```python
from build123d import *

# Parameters (mm, degrees)
BOSS_EXTRUDE1_DEPTH = 10
BOSS_EXTRUDE2_START = 36
BOSS_EXTRUDE2_DEPTH = 36
BOSS_EXTRUDE3_START = 10
BOSS_EXTRUDE3_DEPTH = 10
SKETCH4_R           = 2.5
BOSS_EXTRUDE4_DEPTH = 25
SKETCH4_3_R         = 12.7
BOSS_EXTRUDE5_DEPTH = 2
CUT_EXTRUDE1_START  = -15
CUT_EXTRUDE1_DEPTH  = 15


with BuildPart() as part:
    # Sketch1 → Boss-Extrude1 (new body)
    with BuildSketch(Plane(origin=(0, 0, 0), x_dir=(0, 0, -1), z_dir=(1, 0, 0))):
        with BuildLine():
            Line((-20, 26), (-20, 25))
            ThreePointArc((-20, 25), (-21.464466094, 21.464466094), (-25, 20))
            Line((-25, 20), (-26, 20))
            ThreePointArc((-26, 20), (-27.414213562, 19.414213562), (-28, 18))
            Line((-28, 18), (-28, -18))
            ThreePointArc((-28, -18), (-27.414213562, -19.414213562), (-26, -20))
            Line((-26, -20), (-25, -20))
            ThreePointArc((-25, -20), (-21.464466094, -21.464466094), (-20, -25))
            Line((-20, -25), (-20, -26))
            ThreePointArc((-20, -26), (-19.414213562, -27.414213562), (-18, -28))
            Line((-18, -28), (18, -28))
            ThreePointArc((18, -28), (19.414213562, -27.414213562), (20, -26))
            Line((20, -26), (20, -25))
            ThreePointArc((20, -25), (21.464466094, -21.464466094), (25, -20))
            Line((25, -20), (26, -20))
            ThreePointArc((26, -20), (27.414213562, -19.414213562), (28, -18))
            Line((28, -18), (28, 18))
            ThreePointArc((28, 18), (27.414213562, 19.414213562), (26, 20))
            Line((26, 20), (25, 20))
            ThreePointArc((25, 20), (21.464466094, 21.464466094), (20, 25))
            Line((20, 25), (20, 26))
            ThreePointArc((20, 26), (19.414213562, 27.414213562), (18, 28))
            Line((18, 28), (-18, 28))
            ThreePointArc((-18, 28), (-19.414213562, 27.414213562), (-20, 26))
        make_face()
    extrude(amount=-BOSS_EXTRUDE1_DEPTH)

    # Sketch2 → Boss-Extrude2 (add)
    with BuildSketch(Plane(origin=(0, 0, 0), x_dir=(0, 0, -1), z_dir=(1, 0, 0)).offset(BOSS_EXTRUDE2_START)):
        with BuildLine():
            Line((20, -26), (20, -25))
            ThreePointArc((20, -25), (21.464466094, -21.464466094), (25, -20))
            Line((25, -20), (26, -20))
            ThreePointArc((26, -20), (27.414213562, -19.414213562), (28, -18))
            Line((28, -18), (28, 18))
            ThreePointArc((28, 18), (27.414213562, 19.414213562), (26, 20))
            Line((26, 20), (25, 20))
            ThreePointArc((25, 20), (21.464466094, 21.464466094), (20, 25))
            Line((20, 25), (20, 26))
            ThreePointArc((20, 26), (19.414213562, 27.414213562), (18, 28))
            Line((18, 28), (-18, 28))
            ThreePointArc((-18, 28), (-19.414213562, 27.414213562), (-20, 26))
            Line((-20, 26), (-20, 25))
            ThreePointArc((-20, 25), (-21.464466094, 21.464466094), (-25, 20))
            Line((-25, 20), (-26, 20))
            ThreePointArc((-26, 20), (-27.414213562, 19.414213562), (-28, 18))
            Line((-28, 18), (-28, -18))
            ThreePointArc((-28, -18), (-27.414213562, -19.414213562), (-26, -20))
            Line((-26, -20), (-25, -20))
            ThreePointArc((-25, -20), (-21.464466094, -21.464466094), (-20, -25))
            Line((-20, -25), (-20, -26))
            ThreePointArc((-20, -26), (-19.414213562, -27.414213562), (-18, -28))
            Line((-18, -28), (18, -28))
            ThreePointArc((18, -28), (19.414213562, -27.414213562), (20, -26))
        make_face()
    extrude(amount=-BOSS_EXTRUDE2_DEPTH)

    # Sketch3 → Boss-Extrude3 (add)
    with BuildSketch(Plane(origin=(36, 0, 0), x_dir=(0, 0, -1), z_dir=(1, 0, 0)).offset(BOSS_EXTRUDE3_START)):
        with BuildLine():
            Line((-26, -20), (-25, -20))
            ThreePointArc((-25, -20), (-21.464466094, -21.464466094), (-20, -25))
            Line((-20, -25), (-20, -26))
            ThreePointArc((-20, -26), (-19.414213562, -27.414213562), (-18, -28))
            Line((-18, -28), (18, -28))
            ThreePointArc((18, -28), (19.414213562, -27.414213562), (20, -26))
            Line((20, -26), (20, -25))
            ThreePointArc((20, -25), (21.464466094, -21.464466094), (25, -20))
            Line((25, -20), (26, -20))
            ThreePointArc((26, -20), (27.414213562, -19.414213562), (28, -18))
            Line((28, -18), (28, 18))
            ThreePointArc((28, 18), (27.414213562, 19.414213562), (26, 20))
            Line((26, 20), (25, 20))
            ThreePointArc((25, 20), (21.464466094, 21.464466094), (20, 25))
            Line((20, 25), (20, 26))
            ThreePointArc((20, 26), (19.414213562, 27.414213562), (18, 28))
            Line((18, 28), (-18, 28))
            ThreePointArc((-18, 28), (-19.414213562, 27.414213562), (-20, 26))
            Line((-20, 26), (-20, 25))
            ThreePointArc((-20, 25), (-21.464466094, 21.464466094), (-25, 20))
            Line((-25, 20), (-26, 20))
            ThreePointArc((-26, 20), (-27.414213562, 19.414213562), (-28, 18))
            Line((-28, 18), (-28, -18))
            ThreePointArc((-28, -18), (-27.414213562, -19.414213562), (-26, -20))
        make_face()
    extrude(amount=-BOSS_EXTRUDE3_DEPTH)

    # Sketch4 → Boss-Extrude4 (add)
    with BuildSketch(Plane(origin=(46, 0, 0), x_dir=(0, 0, -1), z_dir=(1, 0, 0))):
        Circle(SKETCH4_R)
    extrude(amount=BOSS_EXTRUDE4_DEPTH)

    # Sketch4<3> → Boss-Extrude5 (add)
    with BuildSketch(Plane(origin=(46, 0, 0), x_dir=(0, 0, -1), z_dir=(1, 0, 0))):
        Circle(SKETCH4_3_R)
    extrude(amount=BOSS_EXTRUDE5_DEPTH)

    # Sketch5 → Cut-Extrude1 (cut)
    with BuildSketch(Plane(origin=(71, 0, 0), x_dir=(0, 0, -1), z_dir=(1, 0, 0)).offset(CUT_EXTRUDE1_START)):
        with BuildLine():
            Line((-2, 1.5), (2, 1.5))
            ThreePointArc((2, 1.5), (0, 2.5), (-2, 1.5))
        make_face()
    extrude(amount=CUT_EXTRUDE1_DEPTH, mode=Mode.SUBTRACT)


solid = part.part
```
Verification items for the finished model (mm, model axes). A direction names the side the tool comes from. Give positions to 0.01 mm unless a question says otherwise; leave off trailing zeros. Write each loop counter-clockwise with the first axis right and the second up, starting at its lowest first coordinate (ties: lowest second). Pieces come first, ordered by that corner, then holes. Notation, with made-up numbers: (-2, 48) - (33, 48) arc R14 ccw to (33, 66) - close; hole circle Ø6 at (2, 70). An arc over 180 degrees is marked (long way). Put each result on its own line as item: value.
Q1. Section check D-D on z = -10.5. Record the cut outline in (x, y).
Result:
outline: (-10, -28) - (46, -28) - (46, -7.14) - (48, -7.14) - (48, 7.14) - (46, 7.14) - (46, 28) - (-10, 28) - close
Q2. Section check B-B on x = -4. Record the cut outline in (y, z), and give its area (3 significant figures).
Result:
outline: (-28, -18) arc R2 ccw to (-26, -20) - (-25, -20) arc R5 cw to (-20, -25) - (-20, -26) arc R2 ccw to (-18, -28) - (18, -28) arc R2 ccw to (20, -26) - (20, -25) arc R5 cw to (25, -20) - (26, -20) arc R2 ccw to (28, -18) - (28, 18) arc R2 ccw to (26, 20) - (25, 20) arc R5 cw to (20, 25) - (20, 26) arc R2 ccw to (18, 28) - (-18, 28) arc R2 ccw to (-20, 26) - (-20, 25) arc R5 cw to (-25, 20) - (-26, 20) arc R2 ccw to (-28, 18) - close
area: 2,890 mm2
Q3. Section check C-C on z = 0. Record the cut outline in (x, y).
Result:
outline: (-10, -28) - (46, -28) - (46, -12.7) - (48, -12.7) - (48, -2.5) - (71, -2.5) - (71, 1.5) - (56, 1.5) - (56, 2.5) - (48, 2.5) - (48, 12.7) - (46, 12.7) - (46, 28) - (-10, 28) - close
Q4. Scan lines: probe 1 along X at (y, z) = (-17, 15.5); probe 2 along X at (y, z) = (-2, -6.5); probe 3 along Y at (x, z) = (51.5, 0). Record each from-to range of solid material in increasing order. Write a range as from..to.
Result:
probe 1: -10..46
probe 2: -10..48
probe 3: -2.5..2.5
Q5. Section check A-A on y = 0. Record the cut outline in (x, z), and give its area (3 significant figures).
Result:
outline: (-10, -28) - (46, -28) - (46, -12.7) - (48, -12.7) - (48, -2.5) - (71, -2.5) - (71, 2.5) - (48, 2.5) - (48, 12.7) - (46, 12.7) - (46, 28) - (-10, 28) - close
area: 3,300 mm2
Q6. Depth check by flat-ended pin: P1, Ø1.1, axis at x = 17, z = -25.5, coming from the +Y side; P2, Ø0.8, axis at x = 20, z = 25.5, coming from the -Y side; P3, Ø1.2, axis at x = 67, z = 0, coming from the +Y side. Enter the tip coordinate at first touch or a pass-through.
Result:
P1: y = 20
P2: y = -20
P3: y = 1.5
Q7. Set-up check for faces 1 (the face through (18, 28, 0)), 2 (the face through (63, 1.5, 0)), 3 (the face through (46, 0, 13)): record each of +Z, -Z, +X, -X, +Y, -Y from which the full face is reachable in a straight line by a thin tool's end or side.
Result:
face 1: +Z, -Z, +X, -X, +Y
face 2: +Z, -Z, +X, +Y
face 3: +X
